```python
from build123d import *

# Parameters (mm, degrees)
SKETCH1_W           = 26
SKETCH1_H           = 40
BOSS_EXTRUDE1_DEPTH = 40
SKETCH2_W           = 26
SKETCH2_H           = 3.7
BOSS_EXTRUDE2_DEPTH = 16
SKETCH5_W           = 20
SKETCH5_H           = 34
CUT_EXTRUDE3_DEPTH  = 37
FILLET1_R           = 1
FILLET2_R           = 1
CUT_EXTRUDE6_DEPTH  = 3.5
SKETCH9_W           = 26
SKETCH9_H           = 1
BOSS_EXTRUDE3_DEPTH = 2
CUT_EXTRUDE7_REACH  = 62.652
SKETCH12_R          = 2.1
CUT_EXTRUDE8_REACH  = 51.947
SKETCH13_R          = 2.1
FILLET3_R           = 2


with BuildPart() as part:
    # Sketch1 → Boss-Extrude1 (new body)
    with BuildSketch(Plane(origin=(0, 0, 0), x_dir=(1, 0, 0), z_dir=(0, 1, 0))):
        Rectangle(SKETCH1_W, SKETCH1_H)
    extrude(amount=BOSS_EXTRUDE1_DEPTH)

    # Sketch2 → Boss-Extrude2 (add)
    with BuildSketch(Plane.XZ):
        with Locations((0, 21.85)):
            Rectangle(SKETCH2_W, SKETCH2_H)
        with Locations((0, -21.85)):
            Rectangle(SKETCH2_W, SKETCH2_H)
    extrude(amount=-BOSS_EXTRUDE2_DEPTH)

    # Sketch5 → Cut-Extrude3 (cut)
    with BuildSketch(Plane.XZ):
        Rectangle(SKETCH5_W, SKETCH5_H)
    extrude(amount=-CUT_EXTRUDE3_DEPTH, mode=Mode.SUBTRACT)

    # Fillet1
    fillet1_edges = [part.edges().sort_by_distance(p)[0] for p in [
        (13, 40, 0),
        (0, 40, -20),
        (-13, 16, 21.85),
        (13, 16, 21.85),
        (0, 16, 20),
        (-13, 16, -21.85),
        (0, 16, -20),
        (13, 16, -21.85),
        (-13, 40, 0),
        (0, 40, 20),
        (-13, 28, -20),
        (13, 28, -20),
        (13, 28, 20),
        (-13, 28, 20),
    ]]
    fillet(fillet1_edges, radius=FILLET1_R)

    # Fillet2
    fillet2_edges = [part.edges().sort_by_distance(p)[0] for p in [
        (-10, 37, 0),
        (-10, 18.5, -17),
        (0, 37, 17),
        (-10, 18.5, 17),
        (10, 37, 0),
        (10, 18.5, 17),
        (0, 37, -17),
        (10, 18.5, -17),
    ]]
    fillet(fillet2_edges, radius=FILLET2_R)

    # Sketch3 → Cut-Extrude6 (cut)
    with BuildSketch(Plane(origin=(0, 0, -23.7), x_dir=(-1, 0, 0), z_dir=(0, 0, -1))):
        Polygon((2.078460969, 11.6), (-2.078460969, 11.6), (-4.156921938, 8), (-2.078460969, 4.4), (2.078460969, 4.4), (4.156921938, 8), align=None)
    cut_extrude6 = extrude(amount=-CUT_EXTRUDE6_DEPTH, mode=Mode.SUBTRACT)

    # Mirror2: Cut-Extrude6 across plane
    add(cut_extrude6.mirror(Plane.XY), mode=Mode.SUBTRACT)

    # Sketch9 → Boss-Extrude3 (add)
    with BuildSketch(Plane.XZ):
        with Locations((0, 20.7)):
            Rectangle(SKETCH9_W, SKETCH9_H)
        with Locations((0, -20.7)):
            Rectangle(SKETCH9_W, SKETCH9_H)
    extrude(amount=BOSS_EXTRUDE3_DEPTH)

    # Sketch12 → Cut-Extrude7 (cut, up to next)
    with BuildSketch(Plane.XY.offset(20), mode=Mode.PRIVATE) as cut_extrude7_sk1:
        with Locations((0, 24)):
            Circle(SKETCH12_R)
    cut_extrude7_tool1 = extrude(cut_extrude7_sk1.sketch, amount=-CUT_EXTRUDE7_REACH, mode=Mode.PRIVATE) & part.part
    add(cut_extrude7_tool1.solids().sort_by_distance((0, 24, 20))[0], mode=Mode.SUBTRACT)

    # Sketch13 → Cut-Extrude8 (cut, up to next)
    with BuildSketch(Plane(origin=(0, 40, 0), x_dir=(1, 0, 0), z_dir=(0, 1, 0)), mode=Mode.PRIVATE) as cut_extrude8_sk1:
        with Locations(Location((0, 10, 0), (0, 0, 270))):
            Circle(SKETCH13_R)
    cut_extrude8_tool1 = extrude(cut_extrude8_sk1.sketch, amount=-CUT_EXTRUDE8_REACH, mode=Mode.PRIVATE) & part.part
    add(cut_extrude8_tool1.solids().sort_by_distance((0, 40, -10))[0], mode=Mode.SUBTRACT)

    # Fillet3
    fillet3_edges = [part.edges().sort_by_distance(p)[0] for p in [
        (0, 0, 21.2),
        (0, 0, -21.2),
    ]]
    fillet(fillet3_edges, radius=FILLET3_R - 0.0001)  # a hair under: the kernel refuses the full size


solid = part.part
```
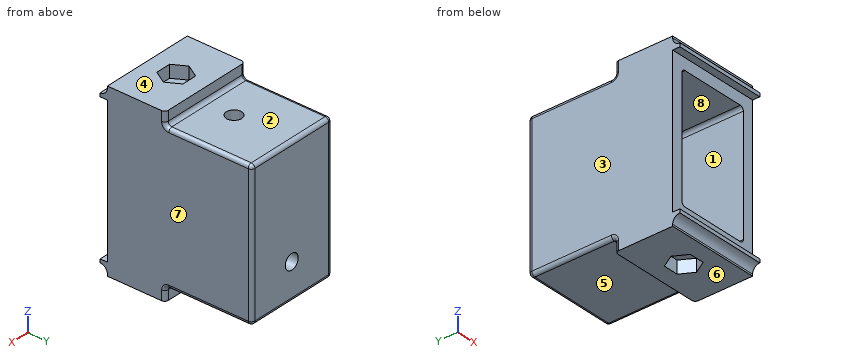
Here's how the part is built. I have some questions about the finished solid (model axes, mm). Face numbers are marked on the shaded views. A direction names the side the tool comes from. Round coordinates to 2 decimals unless told otherwise and drop trailing zeros. Loops run counter-clockwise (first coordinate to the right, second up) from the corner with the lowest first, then second, coordinate; pieces in that order, holes last. Notation, with made-up numbers: (-12, 2) -> (16, 2) arc R10 ccw to (16, 13) -> close; hole circle Ø10 at (-9, 88.25). An arc over 180 degrees is marked (long way). Answer as CSV lines item,"result". Start each with the question number.
1. I'm going to push flat-ended pins straight in: P1, Ø3, axis at x = 6, z = -18, coming from the -Y side; P2, Ø1.8, axis at x = -1, z = -22, coming from the +Y side; P3, Ø1.6, axis at x = 2, y = -1, coming from the -Z side. Where does each tip first touch, or does it pass through?
2. For the marked faces 1, 2, 3, 4 and 5, which set-ups out of +Z, -Z, +X, -X, +Y, -Y let a thin tool reach every point of the face, with its end or its side?
3. Imagine slicing it at D-D on x = 0. State how many separate pieces and enclosed holes the cut face has, plus the area to 3 significant figures.
4. Imagine slicing it at C-C on z = 9.5. Write out the boundary of the cut face in (x, y), plus the area to 3 significant figures.
5. If we mould it in two halves opening along Z, with no side actions, what happens to the marked faces 6, 7 and 8? For each: pulls with the +Z half, pulls with the -Z half, needs draft (parallel to the pull), parting line crosses it, or undercut.
6. I need wall thicknesses on probe 1 along X at (y, z) = (10, 4.5); probe 2 along Y at (x, z) = (0, 18.5); probe 3 along Z at (x, y) = (7.75, 26.5). Which ranges of each line are inside material? Lowest first, please. Write a range as from..to.
7. Imagine slicing it at B-B on y = 1.5. Write out the boundary of the cut face in (x, z).
8. Imagine slicing it at A-A on z = -10. Write out the boundary of the cut face in (x, y), plus the area to 3 significant figures.
Solution:
1,P1,"y = 0"
1,P2,"y = 16"
1,P3,"z = -22.33"
2,face 1,"-Y"
2,face 2,"+Z, +X, -X, +Y"
2,face 3,"+Z, -Z, -X, +Y, -Y"
2,face 4,"+Z, +X, -X, +Y, -Y"
2,face 5,"-Z, +X, -X, +Y"
3,separate pieces,"3"
3,enclosed holes,"0"
3,area,"391 mm²"
4,outline,"(-13, 0) -> (-10, 0) -> (-10, 36) arc R1 cw to (-9, 37) -> (9, 37) arc R1 cw to (10, 36) -> (10, 0) -> (13, 0) -> (13, 39) arc R1 ccw to (12, 40) -> (-12, 40) arc R1 ccw to (-13, 39) -> close"
4,area,"300 mm²"
5,face 6,"pulls with the -Z half"
5,face 7,"needs draft"
5,face 8,"undercut"
6,probe 1,"-13..-10, 10..13"
6,probe 2,"0..21.9, 26.1..40"
6,probe 3,"-20..-17, 17..20"
7,outline,"(-13, -23.7) -> (13, -23.7) -> (13, 23.7) -> (-13, 23.7) -> close; hole (-10, -16) arc R1 ccw to (-9, -17) -> (9, -17) arc R1 ccw to (10, -16) -> (10, 16) arc R1 ccw to (9, 17) -> (-9, 17) arc R1 ccw to (-10, 16) -> close"
8,outline,"(-13, 0) -> (-10, 0) -> (-10, 36) arc R1 cw to (-9, 37) -> (-2.1, 37) -> (-2.1, 40) -> (-12, 40) arc R1 ccw to (-13, 39) -> close; (2.1, 37) -> (9, 37) arc R1 cw to (10, 36) -> (10, 0) -> (13, 0) -> (13, 39) arc R1 ccw to (12, 40) -> (2.1, 40) -> close"
8,area,"287 mm²"
